Geometry: final body of the model. Coordinates: model frame, mm. A direction names the side the tool comes from. Give positions to 0.01 mm unless a question says otherwise; leave off trailing zeros. Write each loop counter-clockwise with the first axis right and the second up, starting at its lowest first coordinate (ties: lowest second). Pieces come first, ordered by that corner, then holes.
Q1. Cut plane C-C on z = 28. Return the cut outline in (x, y).
Q2. Draft query along X for faces 4 (the face through (2.5, 7, 43)), 5 (the face through (4.57, 7.167, 51.986)), 6 (the face through (0, 0, 0)). Return one class per face: pulls with the +X half, pulls with the -X half, needs draft (parallel to the pull), parting line crosses it, or undercut.
Q3. Line query: L1, parallel to Z at x = -0.75, y = 7.5; L2, parallel to Y at x = 5, z = 38.5; L3, parallel to X at y = 5.5, z = 11.5. Output: solid intervals per line, ascending.
Q4. Pin query (flat end, axial travel): pin 1 (2 mm diameter, centred on y = 7.5, z = 43.5, fed in from -X); pin 2 (2 mm diameter, centred on x = 4, z = 31, fed in from +Y); pin 3 (1.5 mm diameter, centred on x = -1, z = 43, fed in from +Y). Return the tip coordinate at first contact, or that it passes through.
Q5. Cut plane A-A on x = 0. Return the cut outline in (y, z), plus the area to 3 significant figures.
Q6. Reachability of faces 1 (the face through (1.756, -7.907, 50.493)), 2 (the face through (0, 7, 35)), 3 (the face through (-1.84, -8.3, 24.65)) from +Z, -Z, +X, -X, +Y, -Y: full face, straight path, thin tool, end or side. Return the list, or none.
Q7. Cut plane B-B on y = -6.25. Return the cut outline in (x, z), plus the area to 3 significant figures.
Q8. Cut plane D-D on x = -6. Return the cut outline in (y, z).
```python
from build123d import *

# Parameters (mm, degrees)
SKETCH1_R           = 8.5
BOSS_EXTRUDE1_DEPTH = 50
SKETCH2_W           = 5
SKETCH2_H           = 3
CUT_EXTRUDE1_DEPTH  = 15
SKETCH3_R           = 8.5
BOSS_EXTRUDE2_DEPTH = 3
SKETCH4_R           = 9
SKETCH4_R_2         = 8.1
CUT_EXTRUDE2_DEPTH  = 1


with BuildPart() as part:
    # Sketch1 → Boss-Extrude1 (new body)
    with BuildSketch(Plane.XY):
        Circle(SKETCH1_R)
    extrude(amount=BOSS_EXTRUDE1_DEPTH)

    # Sketch2 → Cut-Extrude1 (cut)
    with BuildSketch(Plane.XY.offset(50)):
        with Locations((0, 7)):
            Rectangle(SKETCH2_W, SKETCH2_H)
    extrude(amount=-CUT_EXTRUDE1_DEPTH, mode=Mode.SUBTRACT)

    # Sketch3 → Boss-Extrude2 (add)
    with BuildSketch(Plane.XY.offset(50)):
        Circle(SKETCH3_R)
    extrude(amount=BOSS_EXTRUDE2_DEPTH)

    # Sketch4 → Cut-Extrude2 (cut)
    with BuildSketch(Plane(origin=(0, 0, 50), x_dir=(-1, 0, 0), z_dir=(0, 0, -1))):
        Circle(SKETCH4_R)
        Circle(SKETCH4_R_2, mode=Mode.SUBTRACT)
    extrude(amount=-CUT_EXTRUDE2_DEPTH, mode=Mode.SUBTRACT)


solid = part.part
```
Data:
1. outline: circle Ø17 at (0, 0)
2. face 4: undercut
2. face 5: parting line crosses it
2. face 6: needs draft
3. L1: z = 0 to 35, 50 to 53
3. L2: y = -6.87 to 6.87
3. L3: x = -6.48 to 6.48
4. pin 1: stops at x = -5.48
4. pin 2: stops at y = 7.95
4. pin 3: stops at y = 5.5
5. outline: (-8.5, 0) - (8.5, 0) - (8.5, 35) - (5.5, 35) - (5.5, 50) - (8.1, 50) - (8.1, 51) - (8.5, 51) - (8.5, 53) - (-8.5, 53) - (-8.5, 51) - (-8.1, 51) - (-8.1, 50) - (-8.5, 50) - close
5. area: 855 mm2
6. face 1: none
6. face 2: +Y
6. face 3: +Z, -Z
7. outline: (-5.76, 0) - (5.76, 0) - (5.76, 50) - (5.15, 50) - (5.15, 51) - (5.76, 51) - (5.76, 53) - (-5.76, 53) - (-5.76, 51) - (-5.15, 51) - (-5.15, 50) - (-5.76, 50) - close
7. area: 609 mm2
8. outline: (-6.02, 0) - (6.02, 0) - (6.02, 50) - (5.44, 50) - (5.44, 51) - (6.02, 51) - (6.02, 53) - (-6.02, 53) - (-6.02, 51) - (-5.44, 51) - (-5.44, 50) - (-6.02, 50) - close
